Part model, mm, in its own coordinate system. A direction names the side the tool comes from. Coordinates: 2 decimals unless noted, no trailing zeros. Loops run counter-clockwise (first coordinate to the right, second up) from the corner with the lowest first, then second, coordinate; pieces in that order, holes last. Notation, with made-up numbers: (76, 28.5) - (98, 28.5) arc R26 ccw to (98, 52.5) - close; hole circle Ø5 at (66, 2.5). An arc over 180 degrees is marked (long way). Use a Markdown table: item, result. Add a question column.
1) Pull direction X, two halves, no side cores. Call faces 6 (the face through (31.637, 116.753, 8.631)), 7 (the face through (31, 109.358, -1)), 8 (the face through (-15.604, 117.671, -0.291)): +X half, -X half, draft (parallel to the pull), parting line (faces both ways), or undercut.
2) Band-saw the part on B-B (z = -2.5). Give the cut face in (x, y), plus the area to 3 significant figures.
3) Band-saw the part on C-C (x = -7.5). Give the cut face in (y, z), plus the area to 3 significant figures.
4) Band-saw the part on A-A (y = 117.5). Give the cut face in (x, z).
5) Drop flat-ended pins along their axis: P1, Ø4.5, axis at y = 137.5, z = 0, coming from the -X side; P2, Ø1, axis at y = 131.5, z = -6, coming from the +X side; P3, Ø12, axis at y = 131.5, z = 4.5, coming from the +X side. Give the stop position or say it passes through.
6) Tool access for faces 1 (the face through (-16, 134.568, 0)), 2 (the face through (-10.47, 116.777, 21.813)), 3 (the face through (-10.47, 116.777, -21.813)), 4 (the face through (-7.534, 127.741, -0.551)), 5 (the face through (4.36, 116.753, 10.082)): list every direction of +Z, -Z, +X, -X, +Y, -Y with a clear straight run to the whole face (end or side of a thin tool).
7) Probe probe 1 along Y at (x, z) = (4, -7.5); probe 2 along Y at (x, z) = (-10.5, -11.5); probe 3 along Y at (x, z) = (4, 32). List the from-to ranges inside material, lowest first. Write a range as [from, to].
8) Band-saw the part on D-D (z = 8). Give the cut face in (x, y), plus the area to 3 significant figures.
Autodesk Inventor part; units mm, degrees
ref_plane "YZ Plane" through (0, 0, 0) normal (1, 0, 0) x (0, 1, 0)
ref_plane "XZ Plane" through (0, 0, 0) normal (0, 1, 0) x (-1, 0, 0)
ref_plane "XY Plane" through (0, 0, 0) normal (0, 0, 1) x (1, 0, 0)
ref_plane "Work Plane1" through (0, 0, 0) normal (0, 0, 1) x (1, 0, 0)
sketch "Sketch1" plane through (0, 0, 0) normal (0, 0, 1) x (1, 0, 0)
  line L0 (-38.0834, 109.3576) -> (68.9757, 109.3576)
  line L1 (-38.0834, 138.5676) -> (68.9757, 138.5676)
  line L2 (68.4541, 109.3576) -> (43.944, 138.5676)
  line L3 (68.4541, 109.3576) -> (106.585, 109.3576) construction
  line L4 (-18.3608, 138.5676) -> (-18.3608, 134.5676)
  line L5 (-18.3608, 134.5676) -> (-14.3608, 134.5676)
  line L6 (-14.3608, 134.5676) -> (10.8492, 109.3576)
  point P0 (0, 0)
  dimension "d0" = 29.21
  dimension "d1" = 130
  dimension "d2" = 4
  dimension "d3" = 4
extrude "Extrusion1" add sketch "Sketch1" along normal mid plane 78.6511
sketch "Sketch2" plane through (0, 0, 0) normal (0, 0, 1) x (1, 0, 0)
  line L0 (-38.0834, 109.3576) -> (68.9757, 109.3576)
  line L1 (10.8492, 109.3576) -> (-14.3608, 134.5676)
  line L2 (-5.5484, 125.7552) -> (-25.9454, 109.3576)
  point P0 (0, 0)
extrude "Extrusion2" add sketch "Sketch2" along normal mid plane 45.7835
chamfer "Chamfer1" distance 28.575 angle 40 1 edges at (12.7916, 138.5676, -39.3255) measured on face at (41.0824, 119.0943, -39.3256)
chamfer "Chamfer2" distance 28.575 angle 40 1 edges at (12.7916, 138.5676, 39.3255) measured on face at (41.0824, 119.0943, 39.3256)
chamfer "Chamfer3" distance 7.9375 angle 15 1 edges at (-15.7469, 117.5564, -22.8918) measured on face at (-6.8815, 114.8235, -22.8918)
chamfer "Chamfer4" distance 7.9375 angle 15 1 edges at (-15.7469, 117.5564, 22.8918) measured on face at (-6.8815, 114.8235, 22.8918)
sketch "Sketch3" plane through (10.8492, 109.3576, -39.3255) normal (0, -1, 0) x (1, 0, 0)
  circle A0 centre (18.7843, 31.3255) radius 2.1
  circle A1 centre (-6.2157, 31.3255) radius 2.1
  circle A2 centre (-6.2157, 47.3255) radius 2.1
  circle A3 centre (18.7843, 47.3255) radius 2.1
  point P0 (-10.8492, 39.3255)
extrude "Extrusion3" cut sketch "Sketch3" against normal blind 15
properties part number "Head_Fin"
Answer block:
| question | item | result |
|---|---|---|
| 1 | face 6 | undercut |
| 1 | face 7 | draft |
| 1 | face 8 | -X half |
| 2 | outline | (-25.95, 109.36) - (68.45, 109.36) - (43.94, 138.57) - (-18.36, 138.57) - (-18.36, 134.57) - (-14.36, 134.57) - (-5.55, 125.76) - close |
| 2 | area | 2,060 mm2 |
| 3 | outline | (109.36, -22.89) - (114, -22.89) - (124.19, -20.76) - (124.19, 20.76) - (114, 22.89) - (109.36, 22.89) - close; (127.71, -24.46) - (138.57, -15.35) - (138.57, 15.35) - (127.71, 24.46) - close |
| 3 | area | 1,090 mm2 |
| 4 | outline | (-15.82, -20.76) - (-3.15, -22.89) - (2.71, -22.89) - (2.71, -33.03) - (61.62, -33.03) - (61.62, 33.03) - (2.71, 33.03) - (2.71, 22.89) - (-3.15, 22.89) - (-15.82, 20.76) - close; hole circle Ø4.2 at (4.63, -8); hole circle Ø4.2 at (4.63, 8); hole circle Ø4.2 at (29.63, -8); hole circle Ø4.2 at (29.63, 8) |
| 5 | P1 | x = -18.36 |
| 5 | P2 | x = 50.29 |
| 5 | P3 | x = 54.91 |
| 6 | face 1 | +Z, -Z, -X |
| 6 | face 2 | +Z, -X |
| 6 | face 3 | -Z, -X |
| 6 | face 4 | -X |
| 6 | face 5 | -Y |
| 7 | probe 1 | [124.36, 138.57] |
| 7 | probe 2 | [109.36, 121.77], [130.71, 138.57] |
| 7 | probe 3 | [116.21, 118.72] |
| 8 | outline | (-25.95, 109.36) - (2.53, 109.36) - (2.53, 124.36) - (6.73, 124.36) - (6.73, 109.36) - (27.53, 109.36) - (27.53, 124.36) - (31.73, 124.36) - (31.73, 109.36) - (68.45, 109.36) - (43.94, 138.57) - (-18.36, 138.57) - (-18.36, 134.57) - (-14.36, 134.57) - (-5.55, 125.76) - close |
| 8 | area | 1,930 mm2 |
